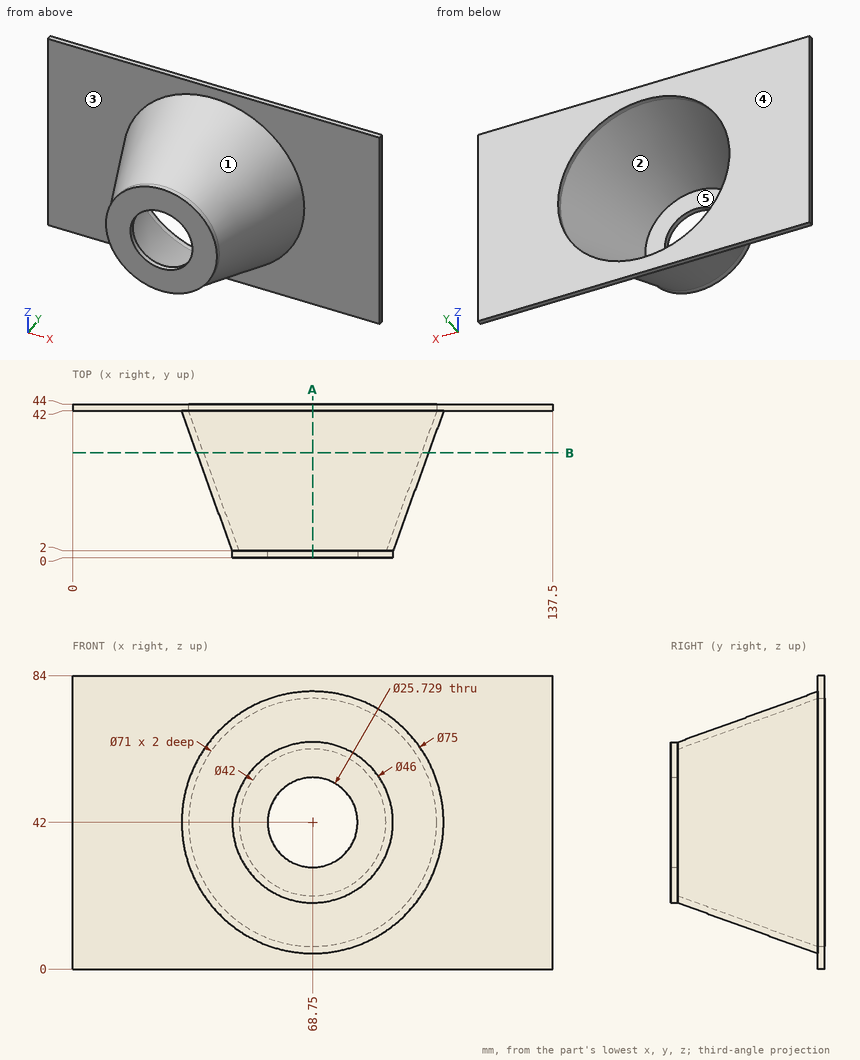
Verification items for this drawing (mm, ordinates from the low corner). A direction names the side the tool comes from. Coordinates: 2 decimals unless noted, no trailing zeros. Order: outer loops, then holes, each group sorted by start corner. A loop starts at its lowest first (then second) coordinate and runs counter-clockwise, first axis right, second up. Notation, with made-up numbers: (-37.75, -0.75) -> (18.25, -0.75) arc R21 cw to (18.25, 37.25) -> close; hole circle Ø2 at (14.25, -15.5). An arc over 180 degrees is marked (long way). Put each result on its own line as item: value. Start each with the question number.
1. Mould release check, pull along Z, two halves, no side actions. Record for the marked faces 1, 2 and 3: released by +Z, released by -Z, zero draft, split by the parting line, or undercut.
2. Go/stop test with flat-tipped pins: pin 1 Ø2 at (x, y) = (79, 30) entering from -Z; pin 2 Ø1 at (x, y) = (78.5, 12) entering from +Z; pin 3 Ø6 at (x, z) = (23.5, 13) entering from -Y. Record where each tip stops, or that it passes through.
3. Material ranges on L1, parallel to Z at x = 68.75, y = 43.45; L2, parallel to Z at x = 68.75, y = 1.15; L3, parallel to Y at x = 130.5, z = 78, recorded low to high. Write a range as [from, to].
4. Cross-section at A-A, the plane x = 68.75. Record the boundary of the cut face in (y, z).
5. Cross-section at B-B, the plane y = 30. Record the boundary of the cut face in (x, z).
6. Access from +Z, -Z, +X, -X, +Y, -Y to the whole of each face (thin tool, end or side, straight path). Record for the marked faces 4 and 5.
Computed:
1. face 1: split by the parting line
1. face 2: undercut
1. face 3: zero draft
2. pin 1: z = 9.98
2. pin 2: z = 67.05
2. pin 3: y = 42
3. L1: [0, 6.5], [77.5, 84]
3. L2: [19, 29.14], [54.86, 65]
3. L3: [42, 44]
4. outline: (0, 19) -> (2, 19) -> (42, 4.5) -> (42, 0) -> (44, 0) -> (44, 6.5) -> (42, 6.5) -> (2, 21) -> (2, 29.14) -> (0, 29.14) -> close; (0, 54.86) -> (2, 54.86) -> (2, 63) -> (42, 77.5) -> (44, 77.5) -> (44, 84) -> (42, 84) -> (42, 79.5) -> (2, 65) -> (0, 65) -> close
5. outline: circle Ø66.3 at (68.75, 42); hole circle Ø62.3 at (68.75, 42)
6. face 4: +Z, -Z, +X, -X, +Y
6. face 5: +Y
